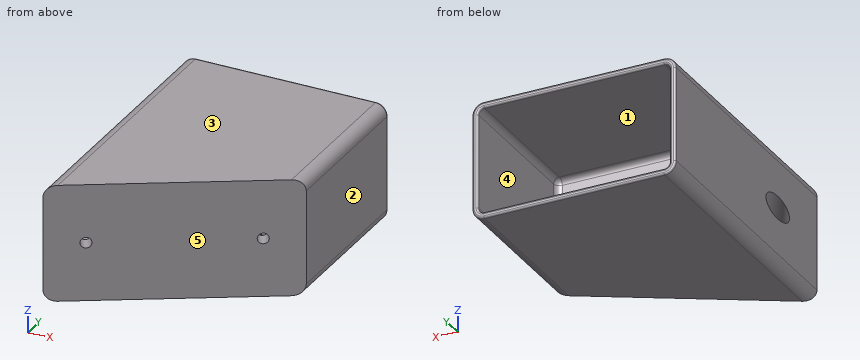
from build123d import *

# Parameters (mm, degrees)
BOSS_EXTRUDE1_DEPTH                                = 27.5
SKETCH3_W                                          = 106
SKETCH3_H                                          = 83
CUT_EXTRUDE1_DEPTH                                 = 28.5
SKETCH4_W                                          = 106
SKETCH4_H                                          = 83
BOSS_EXTRUDE2_DEPTH                                = 3
BOSS_EXTRUDE3_DEPTH                                = 30.5
FILLET1_R                                          = 3
FILLET2_R                                          = 6
FILLET3_R                                          = 1
CUT_EXTRUDE3_START                                 = -10
SKETCH8_R                                          = 6
CUT_EXTRUDE3_DEPTH                                 = 115.880108514
CSK_FOR_10_FLAT_HEAD_MACHINE_SCREW_100_D           = 5.6134
CSK_FOR_10_FLAT_HEAD_MACHINE_SCREW_100_CSINK_D     = 9.779
CSK_FOR_10_FLAT_HEAD_MACHINE_SCREW_100_CSINK_ANGLE = 100


with BuildPart() as part:
    # Sketch1 → Boss-Extrude1 (new body, symmetric)
    with BuildSketch(Plane.XY):
        Polygon((-53, 80), (-50, 80), (-50, 0), (50, 0), (50, 80), (53, 80), (53, -3), (-53, -3), align=None)
    extrude(amount=BOSS_EXTRUDE1_DEPTH, both=True)

    # Sketch3 → Cut-Extrude1 (cut, through all)
    with BuildSketch(Plane.XY):
        with Locations((0, 38.5)):
            Rectangle(SKETCH3_W, SKETCH3_H)
    extrude(amount=-CUT_EXTRUDE1_DEPTH, mode=Mode.SUBTRACT)

    # Sketch4 → Boss-Extrude2 (add)
    with BuildSketch(Plane.XY.offset(27.5)):
        with Locations((0, 38.5)):
            Rectangle(SKETCH4_W, SKETCH4_H)
    extrude(amount=BOSS_EXTRUDE2_DEPTH)

    # Sketch5 → Boss-Extrude3 (add)
    with BuildSketch(Plane.XY.offset(30.5)):
        Polygon((-53, -3), (-53, -64.199128534), (53, -3), align=None)
    extrude(amount=-BOSS_EXTRUDE3_DEPTH)

    # Fillet1
    fillet1_edges = [part.edges().sort_by_distance(p)[0] for p in [
        (-50, 0, 13.75),
        (50, 0, 13.75),
        (50, 40, 27.5),
        (0, 0, 27.5),
        (-50, 40, 27.5),
    ]]
    fillet(fillet1_edges, radius=FILLET1_R)

    # Fillet2
    fillet2_edges = [part.edges().sort_by_distance(p)[0] for p in [
        (-53, 7.900435733, 30.5),
        (53, 38.5, 30.5),
    ]]
    fillet(fillet2_edges, radius=FILLET2_R)

    # Fillet3
    fillet3_edges = [part.edges().sort_by_distance(p)[0] for p in [
        (0, 80, 30.5),
        (-53, 80, 12.25),
        (53, 80, 12.25),
        (51.242640687, 80, 28.742640687),
        (-51.242640687, 80, 28.742640687),
        (0, 80, 27.5),
        (50, 80, 12.25),
        (-50, 80, 12.25),
        (49.121320344, 80, 26.621320344),
        (-49.121320344, 80, 26.621320344),
    ]]
    fillet(fillet3_edges, radius=FILLET3_R)

    # Sketch8 → Cut-Extrude3 (cut, through all)
    with BuildSketch(Plane(origin=(14.549038106, -25.1996732, 0), x_dir=(0.866025404, 0.5, 0), z_dir=(0.5, -0.866025404, 0)).offset(CUT_EXTRUDE3_START)):
        with Locations((-57.998910668, 0)):
            Circle(SKETCH8_R)
        with Locations((24.399346401, 0)):
            Circle(SKETCH8_R)
    extrude(amount=-CUT_EXTRUDE3_DEPTH, mode=Mode.SUBTRACT)

    # CSK for #10 Flat Head Machine Screw (100)2 (through all)
    with Locations(Plane(origin=(-40.679491924, -45.538874496, 0), x_dir=(0.866025404, 0.5, 0), z_dir=(-0.5, 0.866025404, 0))):
        with Locations((0, 0), (82.398257068, 0)):
            CounterSinkHole(CSK_FOR_10_FLAT_HEAD_MACHINE_SCREW_100_D / 2, CSK_FOR_10_FLAT_HEAD_MACHINE_SCREW_100_CSINK_D / 2, counter_sink_angle=CSK_FOR_10_FLAT_HEAD_MACHINE_SCREW_100_CSINK_ANGLE)

    # Mirror1: part across plane


with BuildPart() as part_1:
    add(part.part)
    add(part.part.mirror(Plane.XY))


solid = part_1.part
Input: part model. Units: mm. Frame: model coordinates. Face numbers are marked on the shaded views. A direction names the side the tool comes from. Coordinates: 2 decimals unless noted, no trailing zeros. Order: outer loops, then holes, each group sorted by start corner. A loop starts at its lowest first (then second) coordinate and runs counter-clockwise, first axis right, second up.
1. Access query for the marked faces 4 and 5. Directions: +Z, -Z, +X, -X, +Y, -Y. A direction counts if a zero-diameter tool reaches every point of the face in a straight line with its end or side. Return the directions, or none.
Checked values:
face 4: +Y
face 5: +Z, -Z, +X, -Y
2. Cut plane B-B, the plane z = -11. Return loops of the section in (x, y).
Checked values:
outline: (-53, -64.2) - (53, -3) - (53, 79) arc R1 ccw to (52, 80) - (51, 80) arc R1 ccw to (50, 79) - (50, 3) arc R3 cw to (47, 0) - (-47, 0) arc R3 cw to (-50, 3) - (-50, 79) arc R1 ccw to (-51, 80) - (-52, 80) arc R1 ccw to (-53, 79) - close
3. Cut plane C-C, the plane x = -24. Return loops of the section in (y, z), plus the area to 3 significant figures.
Checked values:
outline: (-47.46, -30.5) - (79, -30.5) arc R1 ccw to (80, -29.5) - (80, -28.5) arc R1 ccw to (79, -27.5) - (3, -27.5) arc R3 cw to (0, -24.5) - (0, 24.5) arc R3 cw to (3, 27.5) - (79, 27.5) arc R1 ccw to (80, 28.5) - (80, 29.5) arc R1 ccw to (79, 30.5) - (-47.46, 30.5) - close
area: 3,380 mm2
4. Draft query along Z for the marked faces 1, 2 and 3. Return one class per face: +Z half, -Z half, draft (parallel to the pull), parting line (faces both ways), or undercut.
Checked values:
face 1: undercut
face 2: draft
face 3: +Z half
5. Cut plane A-A, the plane y = 63. Return loops of the section in (x, z).
Checked values:
outline: (-53, -24.5) arc R6 ccw to (-47, -30.5) - (47, -30.5) arc R6 ccw to (53, -24.5) - (53, 24.5) arc R6 ccw to (47, 30.5) - (-47, 30.5) arc R6 ccw to (-53, 24.5) - close; hole (-50, -24.5) arc R3 ccw to (-47, -27.5) - (47, -27.5) arc R3 ccw to (50, -24.5) - (50, 24.5) arc R3 ccw to (47, 27.5) - (-47, 27.5) arc R3 ccw to (-50, 24.5) - close
6. Contact query for flat-ended pins moving along their axis: P1, Ø8, axis at y = -48, z = -15, coming from the +X side; P2, Ø1, axis at x = -1.5, z = -17.5, coming from the +Y side; P3, Ø5, axis at y = -8.5, z = 19.5, coming from the +X side. Output: stop coordinate, or through.
Checked values:
P1: stops at x = -18.01
P2: stops at y = 0
P3: stops at x = 47.8
7. Ray query, line 1 along X through (y, z) = (42.5, -15.5); line 2 along Z through (x, y) = (-11, 24.5); line 3 along Z through (x, y) = (-2.5, 0.5). Return the intervals inside material, ascending.
Checked values:
line 1: x = -53 to -50, 50 to 53
line 2: z = -30.5 to -27.5, 27.5 to 30.5
line 3: z = -30.5 to -26.16, 26.16 to 30.5
